```python
from build123d import *

# Parameters (mm, degrees)
F1_DEPTH = 5
F2_DEPTH = 50
F3_DEPTH = 2.5


with BuildPart() as f1:
    # F0 (on Front) → F1 (new body, symmetric)
    with BuildSketch(Plane.XZ):
        with BuildLine():
            ThreePointArc((2.5, 10), (2.4800742407, 10.3150107312), (2.4206145914, 10.625))
            ThreePointArc((2.4206145914, 10.625), (0, 12.5), (-2.4206145914, 10.625))
            ThreePointArc((-2.4206145914, 10.625), (-0.3150107312, 7.5199257593), (2.5, 10))
        make_face()
        with BuildLine():
            ThreePointArc((-4.8412291828, 1.25), (0, 5), (4.8412291828, 1.25))
            Line((4.8412291828, 1.25), (2.4206145914, 10.625))
            ThreePointArc((2.4206145914, 10.625), (2.4800742407, 10.3150107312), (2.5, 10))
            ThreePointArc((2.5, 10), (-0.3150107312, 7.5199257593), (-2.4206145914, 10.625))
            Line((-2.4206145914, 10.625), (-4.8412291828, 1.25))
        make_face()
        with BuildLine():
            ThreePointArc((-4.8412291828, 1.25), (-0.6300214624, -4.9601484813), (5, 0))
            ThreePointArc((5, 0), (4.9601484813, 0.6300214624), (4.8412291828, 1.25))
            ThreePointArc((4.8412291828, 1.25), (0, 5), (-4.8412291828, 1.25))
        make_face()
    extrude(amount=F1_DEPTH, both=True)

    # F0 (on Front) → F2 (join, symmetric)
    with BuildSketch(Plane.XZ):
        with BuildLine():
            ThreePointArc((-4.8412291828, 1.25), (-0.6300214624, -4.9601484813), (5, 0))
            ThreePointArc((5, 0), (4.9601484813, 0.6300214624), (4.8412291828, 1.25))
            ThreePointArc((4.8412291828, 1.25), (0, 5), (-4.8412291828, 1.25))
        make_face()
    extrude(amount=F2_DEPTH, both=True)

    # F0 (on Front) → F3 (cut, symmetric)
    with BuildSketch(Plane.XZ):
        with BuildLine():
            ThreePointArc((-4.8412291828, 1.25), (0, 5), (4.8412291828, 1.25))
            Line((4.8412291828, 1.25), (2.4206145914, 10.625))
            ThreePointArc((2.4206145914, 10.625), (2.4800742407, 10.3150107312), (2.5, 10))
            ThreePointArc((2.5, 10), (-0.3150107312, 7.5199257593), (-2.4206145914, 10.625))
            Line((-2.4206145914, 10.625), (-4.8412291828, 1.25))
        make_face()
        with BuildLine():
            ThreePointArc((-4.8412291828, 1.25), (-0.6300214624, -4.9601484813), (5, 0))
            ThreePointArc((5, 0), (4.9601484813, 0.6300214624), (4.8412291828, 1.25))
            ThreePointArc((4.8412291828, 1.25), (0, 5), (-4.8412291828, 1.25))
        make_face()
    extrude(amount=F3_DEPTH, both=True, mode=Mode.SUBTRACT)


solid = f1.part
```
Verification items for the finished model (mm, model axes). Round coordinates to 2 decimals unless told otherwise and drop trailing zeros. Order: outer loops, then holes, each group sorted by start corner. A loop starts at its lowest first (then second) coordinate and runs counter-clockwise, first axis right, second up.
1) Draft check along Y on faces 1 (the flat face through (0, -50, 0)), 2 (the flat face through (0, 50, 0)), 3 (the flat face through (0, 2.5, 1)). Enter one of: +Y half, -Y half, draft (parallel to the pull), parting line (faces both ways), or undercut.
Geometry says:
face 1: -Y half
face 2: +Y half
face 3: undercut
2) Cross-section at B-B, the plane x = -3.75. Record the cut outline in (y, z).
Geometry says:
outline: (-50, -3.31) - (-2.5, -3.31) - (-2.5, 5.48) - (-5, 5.48) - (-5, 3.31) - (-50, 3.31) - close; (2.5, -3.31) - (50, -3.31) - (50, 3.31) - (5, 3.31) - (5, 5.48) - (2.5, 5.48) - close
3) Depth check by flat-ended pin: pin 1 (4 mm diameter, centred on x = -2.5, y = 23.5, fed in from -Z); pin 2 (2 mm diameter, centred on x = 3, y = -6.5, fed in from +Z); pin 3 (1.5 mm diameter, centred on x = -4, y = 17.5, fed in from +Z). Enter the tip coordinate at first touch or a pass-through.
Geometry says:
pin 1: stops at z = -4.97
pin 2: stops at z = 4.58
pin 3: stops at z = 3.8
4) Cross-section at A-A, the plane z = 3. Record the cut outline in (x, y).
Geometry says:
outline: (-4.39, -5) - (-4, -5) - (-4, -50) - (4, -50) - (4, -5) - (4.39, -5) - (4.39, -2.5) - (-4.39, -2.5) - close; (-4.39, 2.5) - (4.39, 2.5) - (4.39, 5) - (4, 5) - (4, 50) - (-4, 50) - (-4, 5) - (-4.39, 5) - close
5) Cross-section at C-C, the plane y = -18.5. Record the cut outline in (x, z).
Geometry says:
outline: circle Ø10 at (0, 0)
6) Material ranges on line 1 (Y direction, x = -1.75, z = -0.75); line 2 (Y direction, x = 3, z = 5); line 3 (X direction, y = -43.5, z = 0.25), recorded low to high.
Geometry says:
line 1: y = -50 to -2.5, 2.5 to 50
line 2: y = -5 to -2.5, 2.5 to 5
line 3: x = -4.99 to 4.99
7) Cross-section at D-D, the plane x = 0. Record the cut outline in (y, z).
Geometry says:
outline: (-50, -5) - (-2.5, -5) - (-2.5, 7.5) - (2.5, 7.5) - (2.5, -5) - (50, -5) - (50, 5) - (5, 5) - (5, 12.5) - (-5, 12.5) - (-5, 5) - (-50, 5) - close
